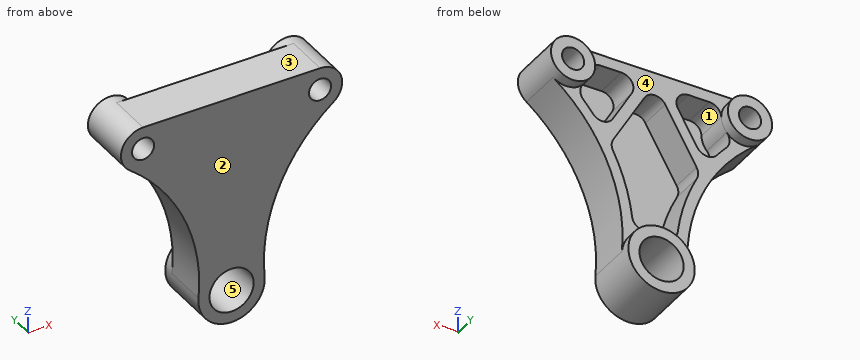
from build123d import *

# Parameters (mm, degrees)
BOSS_EXTRUDE1_DEPTH = 12.7
OUTSIDE_CIRLCES_R   = 9.525
OUTSIDE_CIRLCES_R_2 = 6.35
BOSS_EXTRUDE2_DEPTH = 15.875
SKETCH2_R           = 6.35
SKETCH2_R_2         = 3.175
CUT_EXTRUDE2_DEPTH  = 68.277043819
SHELL1_START        = 3.175
SHELL1_DEPTH        = 9.525
RIB1_START          = -9.525
RIB1_DEPTH          = 9.525
FILLET1_R           = 3.429


# Read off the part's stored shape, not the designer's step: Shell1, Rib1
with BuildPart() as part:
    # Sketch1 → Boss-Extrude1 (new body)
    with BuildSketch(Plane(origin=(0, 0, 0), x_dir=(1, 0, 0), z_dir=(0, 1, 0))):
        with BuildLine():
            Line((-25.4, -57.15), (25.4, -57.15))
            ThreePointArc((25.4, -57.15), (31.415385717, -52.834117665), (29.253859008, -45.753192024))
            ThreePointArc((29.253859008, -45.753192024), (13.590190704, -25.845719106), (9.487062801, -0.849272876))
            ThreePointArc((9.487062801, -0.849272876), (0, 9.525), (-9.487062801, -0.849272876))
            ThreePointArc((-9.487062801, -0.849272876), (-13.590190704, -25.845719106), (-29.253859008, -45.753192024))
            ThreePointArc((-29.253859008, -45.753192024), (-31.415385717, -52.834117665), (-25.4, -57.15))
        make_face()
    extrude(amount=BOSS_EXTRUDE1_DEPTH)

    # Outside Cirlces → Boss-Extrude2 (add)
    with BuildSketch(Plane(origin=(0, 0, 0), x_dir=(1, 0, 0), z_dir=(0, 1, 0))):
        with Locations(Location((0, 0, 0), (0, 0, 354.884571445))):
            Circle(OUTSIDE_CIRLCES_R)
        with Locations(Location((25.4, -50.8, 0), (0, 0, 270))):
            Circle(OUTSIDE_CIRLCES_R_2)
        with Locations(Location((-25.4, -50.8, 0), (0, 0, 90))):
            Circle(OUTSIDE_CIRLCES_R_2)
    extrude(amount=BOSS_EXTRUDE2_DEPTH)

    # Sketch2 → Cut-Extrude2 (cut, through all)
    with BuildSketch(Plane(origin=(0, 0, 0), x_dir=(1, 0, 0), z_dir=(0, 1, 0))):
        with Locations(Location((0, 0, 0), (0, 0, 270))):
            Circle(SKETCH2_R)
        with Locations(Location((-25.4, -50.8, 0), (0, 0, 270))):
            Circle(SKETCH2_R_2)
        with Locations(Location((25.4, -50.8, 0), (0, 0, 270))):
            Circle(SKETCH2_R_2)
    extrude(amount=CUT_EXTRUDE2_DEPTH, mode=Mode.SUBTRACT)

    # Shell1 outline → Shell1 (cut)
    with BuildSketch(Plane(origin=(0, 0, 0), x_dir=(1, 0, 0), z_dir=(0, 1, 0)).offset(SHELL1_START)):
        with BuildLine():
            ThreePointArc((-23.245193613, -44.826783996), (-19.436053982, -48.61966794), (-19.900738686, -53.975))
            Line((-19.900738686, -53.975), (19.900738686, -53.975))
            ThreePointArc((19.900738686, -53.975), (19.436053982, -48.61966794), (23.245193613, -44.826783996))
            ThreePointArc((23.245193613, -44.826783996), (10.964919098, -27.751584466), (6.1431994, -7.279198179))
            ThreePointArc((6.1431994, -7.279198179), (0, -9.525), (-6.1431994, -7.279198179))
            ThreePointArc((-6.1431994, -7.279198179), (-10.964919098, -27.751584466), (-23.245193613, -44.826783996))
        make_face()
    extrude(amount=SHELL1_DEPTH, mode=Mode.SUBTRACT)

    # Rib1 outline → Rib1 (add)
    with BuildSketch(Plane(origin=(0, 12.7, 0), x_dir=(1, 0, 0), z_dir=(0, 1, 0)).offset(RIB1_START)):
        with BuildLine():
            Line((12.912461206, -31.609961141), (0, -53.975))
            Line((0, -53.975), (3.666174209, -53.975))
            Line((3.666174209, -53.975), (14.782281631, -34.721337162))
            ThreePointArc((14.782281631, -34.721337162), (13.82120772, -33.181372554), (12.912461206, -31.609961141))
        make_face()
        with BuildLine():
            Line((0, -53.975), (-12.912461206, -31.609961141))
            ThreePointArc((-12.912461206, -31.609961141), (-13.82120772, -33.181372554), (-14.782281631, -34.721337162))
            Line((-14.782281631, -34.721337162), (-3.666174209, -53.975))
            Line((-3.666174209, -53.975), (0, -53.975))
        make_face()
    extrude(amount=RIB1_DEPTH)

    # Fillet1
    fillet1_edges = [part.edges().sort_by_distance(p)[0] for p in [
        (-12.912461206, 7.9375, 31.609961141),
        (-3.666174209, 7.9375, 53.975),
        (-14.782281631, 7.9375, 34.721337162),
        (14.782281631, 7.9375, 34.721337162),
        (3.666174209, 7.9375, 53.975),
        (0, 7.9375, 53.975),
        (12.912461206, 7.9375, 31.609961141),
        (-6.1431994, 7.9375, 7.279198179),
        (-19.900738686, 7.9375, 53.975),
        (23.245193613, 7.9375, 44.826783996),
        (6.1431994, 7.9375, 7.279198179),
        (-23.245193613, 7.9375, 44.826783996),
        (19.900738686, 7.9375, 53.975),
    ]]
    fillet(fillet1_edges, radius=FILLET1_R)


solid = part.part
Verification items for the finished model (mm, model axes). Face numbers are marked on the shaded views. A direction names the side the tool comes from. Round coordinates to 2 decimals unless told otherwise and drop trailing zeros. Order: outer loops, then holes, each group sorted by start corner. A loop starts at its lowest first (then second) coordinate and runs counter-clockwise, first axis right, second up. Notation, with made-up numbers: (-38.75, -5.5) -> (0.25, -5.5) arc R34 cw to (0.25, 29.5) -> close; hole circle Ø10 at (89.25, 57.25). An arc over 180 degrees is marked (long way). Put each result on its own line as item: value.
1) Section check C-C (x = -17). Record the cut outline in (y, z) (3 decimals), then the cut area to 3 significant figures.
Final values:
outline: (0, 32.292) -> (12.7, 32.292) -> (12.7, 38.182) -> (3.175, 38.182) -> (3.175, 53.687) -> (12.7, 53.687) -> (12.7, 57.15) -> (0, 57.15) -> close
area: 168 mm^2
2) Mould release check, pull along Z, two halves, no side actions. Record for the marked faces 1, 2 and 3: +Z half, -Z half, draft (parallel to the pull), parting line (faces both ways), or undercut.
Final values:
face 1: undercut
face 2: draft
face 3: +Z half
3) Section check A-A (z = 0). Record the cut outline in (x, y) (3 decimals), then the cut area to 3 significant figures.
Final values:
outline: (-9.525, 0) -> (-6.35, 0) -> (-6.35, 15.875) -> (-9.525, 15.875) -> close; (6.35, 0) -> (9.525, 0) -> (9.525, 15.875) -> (6.35, 15.875) -> close
area: 101 mm^2
4) Section check D-D (z = 52). Record the cut outline in (x, y) (1 decimal).
Final values:
outline: (-31.6, 0) -> (-28.3, 0) -> (-28.3, 15.9) -> (-31.6, 15.9) -> close; (-22.5, 0) -> (22.5, 0) -> (22.5, 15.9) -> (19.2, 15.9) -> (19.2, 12.7) -> (18.7, 12.7) -> (18.7, 3.2) -> (6.5, 3.2) -> (6.5, 12.7) -> (-6.5, 12.7) -> (-6.5, 3.2) -> (-18.7, 3.2) -> (-18.7, 12.7) -> (-19.2, 12.7) -> (-19.2, 15.9) -> (-22.5, 15.9) -> close; (28.3, 0) -> (31.6, 0) -> (31.6, 15.9) -> (28.3, 15.9) -> close
5) Set-up check for the marked faces 4 and 5: record each of +Z, -Z, +X, -X, +Y, -Y from which the full face is reachable in a straight line by a thin tool's end or side.
Final values:
face 4: +Y
face 5: +Y, -Y
6) Material ranges on line 1 (X direction, y = 7.25, z = 50.8) (3 decimals); line 2 (X direction, y = 10, z = 43); line 3 (X direction, y = 10.75, z = 46.5), recorded low to high.
Final values:
line 1: x = -31.75 to -28.575, -22.225 to -19.044, -6.186 to 6.186, 19.044 to 22.225, 28.575 to 31.75
line 2: x = -25.95 to -21.12, -10 to -6.34, 6.34 to 10, 21.12 to 25.95
line 3: x = -30.07 to -20.72, -7.98 to -4.32, 4.32 to 7.98, 20.72 to 30.07
7) Depth check by flat-ended pin: pin 1 (2 mm diameter, centred on x = -4, z = 13, fed in from -Y); pin 2 (6 mm diameter, centred on y = 5, z = 39.5, fed in from +X); pin 3 (12.5 mm diameter, centred on x = 0, z = 36, fed in from +Y) (3 decimals); pin 4 (12 mm diameter, centred on x = 12, z = 42.5, fed in from +Y). Enter the tip coordinate at first touch or a pass-through.
Final values:
pin 1: stops at y = 0
pin 2: stops at x = 25.41
pin 3: stops at y = 3.175
pin 4: stops at y = 12.7
8) Section check B-B (y = 14.75). Record the cut outline in (x, z) (3 decimals), then the cut area to 3 significant figures.
Final values:
outline: circle Ø12.7 at (-25.4, 50.8); circle Ø19.05 at (0, 0); circle Ø12.7 at (25.4, 50.8); hole circle Ø6.35 at (-25.4, 50.8); hole circle Ø12.7 at (0, 0); hole circle Ø6.35 at (25.4, 50.8)
area: 348 mm^2
